Design review of the part built by this model. Coordinates are the model's own, in mm. Round coordinates to 2 decimals unless told otherwise and drop trailing zeros. Write each loop counter-clockwise with the first axis right and the second up, starting at its lowest first coordinate (ties: lowest second). Pieces come first, ordered by that corner, then holes. Notation, with made-up numbers: M -7,27 L 13,27 A19 cw 13,40 Z; hole C -1.75,64 d2. An arc over 180 degrees is marked long. Use CSV: the item, a comma, the result in double quotes.
from build123d import *

# Parameters (mm, degrees)
SKETCH_1_W          = 117
SKETCH_1_H          = 80
EXTRUDE_1_DEPTH     = 5
SKETCH_2_R          = 1.525
CUT_EXTRUDE_1_DEPTH = 5
SKETCH_3_R          = 2.025
CUT_EXTRUDE_2_DEPTH = 5
SKETCH_4_R          = 2.025
CUT_EXTRUDE_3_DEPTH = 5
SKETCH_5_R          = 1.525
CUT_EXTRUDE_4_DEPTH = 5
SKETCH_6_R          = 1.525
CUT_EXTRUDE_5_DEPTH = 5
SKETCH_7_R          = 2.024999998
CUT_EXTRUDE_6_DEPTH = 5
SKETCH_9_W          = 117
SKETCH_9_H          = 6
EXTRUDE_2_DEPTH     = 5
FILLET_2_R          = 4
SKETCH_10_W         = 2.1
SKETCH_10_H         = 5.1
SKETCH_10_W_2       = 20.9
CUT_EXTRUDE_7_DEPTH = 5


with BuildPart() as part:
    # 草图1 → 凸台-拉伸1 (new body)
    with BuildSketch(Plane.XY):
        Rectangle(SKETCH_1_W, SKETCH_1_H)
    extrude(amount=EXTRUDE_1_DEPTH)

    # 草图2 → 切除-拉伸1 (cut)
    with BuildSketch(Plane.XY.offset(5)):
        with Locations((-27, -20.55)):
            Circle(SKETCH_2_R)
        with Locations((-42, -20.55)):
            Circle(SKETCH_2_R)
        with Locations((-42, -30.55)):
            Circle(SKETCH_2_R)
        with Locations((-27, -30.55)):
            Circle(SKETCH_2_R)
        with Locations((-42, 27.5)):
            Circle(SKETCH_2_R)
        with Locations((-42, 17.5)):
            Circle(SKETCH_2_R)
        with Locations((-27, 27.5)):
            Circle(SKETCH_2_R)
        with Locations((-27, 17.5)):
            Circle(SKETCH_2_R)
    cut_extrude_1 = extrude(amount=-CUT_EXTRUDE_1_DEPTH, mode=Mode.SUBTRACT)

    # 镜向1: 切除-拉伸1 across plane
    add(cut_extrude_1.mirror(Plane(origin=(0, 0, 0), x_dir=(0, 0, 1), z_dir=(1, 0, 0))), mode=Mode.SUBTRACT)

    # 草图3 → 切除-拉伸2 (cut)
    with BuildSketch(Plane.XY.offset(5)):
        with Locations((-8.5, 21)):
            Circle(SKETCH_3_R)
        with Locations((8.5, 21)):
            Circle(SKETCH_3_R)
        with Locations((8.5, 6)):
            Circle(SKETCH_3_R)
        with Locations((-8.5, 6)):
            Circle(SKETCH_3_R)
    extrude(amount=-CUT_EXTRUDE_2_DEPTH, mode=Mode.SUBTRACT)

    # 草图4 → 切除-拉伸3 (cut)
    with BuildSketch(Plane.XY.offset(5)):
        with Locations((8.5, -17.25)):
            Circle(SKETCH_4_R)
        with Locations((8.5, -32.25)):
            Circle(SKETCH_4_R)
        with Locations((-8.5, -32.25)):
            Circle(SKETCH_4_R)
        with Locations((-8.5, -17.25)):
            Circle(SKETCH_4_R)
    extrude(amount=-CUT_EXTRUDE_3_DEPTH, mode=Mode.SUBTRACT)

    # 草图5 → 切除-拉伸4 (cut)
    with BuildSketch(Plane.XY.offset(5)):
        with Locations((-55.5, -5)):
            Circle(SKETCH_5_R)
        with Locations((-55.5, -25)):
            Circle(SKETCH_5_R)
    cut_extrude_4 = extrude(amount=-CUT_EXTRUDE_4_DEPTH, mode=Mode.SUBTRACT)

    # 镜向2: 切除-拉伸4 across plane
    add(cut_extrude_4.mirror(Plane(origin=(0, 0, 0), x_dir=(0, 0, 1), z_dir=(1, 0, 0))), mode=Mode.SUBTRACT)

    # 草图6 → 切除-拉伸5 (cut)
    with BuildSketch(Plane.XY.offset(5)):
        with Locations((0, 19.85)):
            Circle(SKETCH_6_R)
        with Locations((0, 7.15)):
            Circle(SKETCH_6_R)
        with Locations((0, -18.4)):
            Circle(SKETCH_6_R)
        with Locations((0, -31.1)):
            Circle(SKETCH_6_R)
    extrude(amount=-CUT_EXTRUDE_5_DEPTH, mode=Mode.SUBTRACT)

    # 草图7 → 切除-拉伸6 (cut)
    with BuildSketch(Plane.XY.offset(5)):
        with Locations((26, -4.049999992)):
            Circle(SKETCH_7_R)
        with Locations((11, -4.049999992)):
            Circle(SKETCH_7_R)
    cut_extrude_6 = extrude(amount=-CUT_EXTRUDE_6_DEPTH, mode=Mode.SUBTRACT)

    # 镜向4: 切除-拉伸6 across plane
    add(cut_extrude_6.mirror(Plane(origin=(0, 0, 0), x_dir=(0, 0, 1), z_dir=(1, 0, 0))), mode=Mode.SUBTRACT)

    # 草图9 → 凸台-拉伸2 (add)
    with BuildSketch(Plane.XY.offset(5)):
        with Locations((0, 43)):
            Rectangle(SKETCH_9_W, SKETCH_9_H)
    extrude(amount=-EXTRUDE_2_DEPTH)

    # 圆角2
    fillet_2_edges = [part.edges().sort_by_distance(p)[0] for p in [
        (58.5, 46, 2.5),
        (-58.5, 46, 2.5),
        (58.5, -40, 2.5),
        (-58.5, -40, 2.5),
    ]]
    fillet(fillet_2_edges, radius=FILLET_2_R)

    # 草图10 → 切除-拉伸7 (cut)
    with BuildSketch(Plane.XY.offset(5)):
        with BuildLine():
            ThreePointArc((-36.45, 40.05), (-37.5, 41.1), (-38.55, 40.05))
            Line((-38.55, 40.05), (-36.45, 40.05))
        make_face()
        with Locations((-37.5, 37.5)):
            Rectangle(SKETCH_10_W, SKETCH_10_H)
        with Locations((-26, 37.5)):
            Rectangle(SKETCH_10_W_2, SKETCH_10_H)
        with BuildLine():
            Line((-36.45, 34.95), (-38.55, 34.95))
            ThreePointArc((-38.55, 34.95), (-37.5, 33.9), (-36.45, 34.95))
        make_face()
        with BuildLine():
            ThreePointArc((-13.45, 40.05), (-14.5, 41.1), (-15.55, 40.05))
            Line((-15.55, 40.05), (-13.45, 40.05))
        make_face()
        with Locations((-14.5, 37.5)):
            Rectangle(SKETCH_10_W, SKETCH_10_H)
        with BuildLine():
            Line((-13.45, 34.95), (-15.55, 34.95))
            ThreePointArc((-15.55, 34.95), (-14.5, 33.9), (-13.45, 34.95))
        make_face()
    cut_extrude_7 = extrude(amount=-CUT_EXTRUDE_7_DEPTH, mode=Mode.SUBTRACT)

    # 镜向5: 切除-拉伸7 across plane
    add(cut_extrude_7.mirror(Plane(origin=(0, 0, 0), x_dir=(0, 0, 1), z_dir=(1, 0, 0))), mode=Mode.SUBTRACT)


solid = part.part
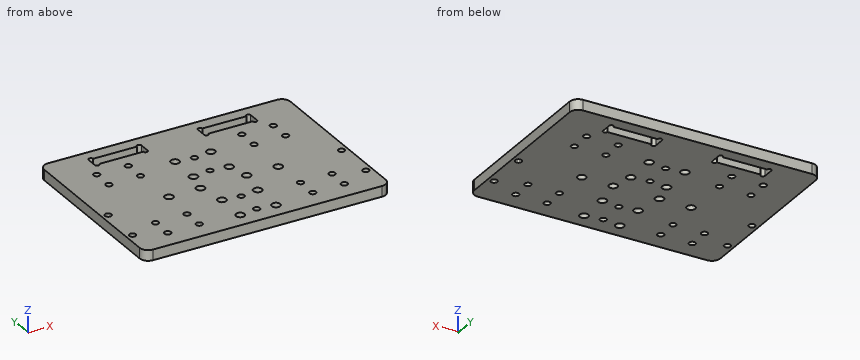
1) Add section B-B on z = 3.1. Give the number of separate pieces and of enclosed holes in the cut face, then the cut area to 3 significant figures.
Answers:
separate pieces,"1"
enclosed holes,"38"
area,"9,450 mm²"
2) Add section A-A on x = 0. Write out the cut boundary in (y, z) (3 decimals).
Answers:
outline,"M -40,0 L -32.625,0 L -32.625,5 L -40,5 Z; M -29.575,0 L -19.925,0 L -19.925,5 L -29.575,5 Z; M -16.875,0 L 5.625,0 L 5.625,5 L -16.875,5 Z; M 8.675,0 L 18.325,0 L 18.325,5 L 8.675,5 Z; M 21.375,0 L 46,0 L 46,5 L 21.375,5 Z"
3) Wall thickness on line 1 along Y through (x, z) = (8.5, 1.2) (3 decimals); line 2 along Y through (x, z) = (42, 1.55) (3 decimals); line 3 along X through (y, z) = (38, 2.5): over which ranges is each line inside the solid? List them lowest first. Write a range as [from, to].
Answers:
line 1,"[-40, -34.275], [-30.225, -19.275], [-15.225, 3.975], [8.025, 18.975], [23.025, 46]"
line 2,"[-40, -32.075], [-29.025, -22.075], [-19.025, 15.975], [19.025, 25.975], [29.025, 46]"
line 3,"[-58.5, -38.55], [-13.45, 13.45], [38.55, 58.5]"
